from build123d import *

# Parameters (mm, degrees)
BOSS_EXTRUDE2_DEPTH = 6.35
SKETCH2_R           = 3.175
CUT_EXTRUDE1_DEPTH  = 7.35
SKETCH7_R           = 2.286
CUT_EXTRUDE3_DEPTH  = 12.7
SKETCH8_R           = 2.286
CUT_EXTRUDE4_DEPTH  = 7.35
SKETCH9_W           = 129.404437756
SKETCH9_H           = 25.4
CUT_EXTRUDE5_DEPTH  = 7.35
CUT_EXTRUDE6_DEPTH  = 3.175
BOSS_EXTRUDE3_DEPTH = 3.81
CHAMFER1_SIZE       = 2.54


with BuildPart() as part:
    # Sketch1 → Boss-Extrude2 (new body)
    with BuildSketch(Plane(origin=(0, 0, 0), x_dir=(1, 0, 0), z_dir=(0, 1, 0))):
        with BuildLine():
            Line((0, 0), (0, 25.4))
            ThreePointArc((0, 25.4), (3.719743879, 34.380256121), (12.7, 38.1))
            Line((12.7, 38.1), (190.5, 38.1))
            ThreePointArc((190.5, 38.1), (199.480256121, 34.380256121), (203.2, 25.4))
            Line((203.2, 25.4), (203.2, -152.4))
            ThreePointArc((203.2, -152.4), (199.480256121, -161.380256121), (190.5, -165.1))
            Line((190.5, -165.1), (12.7, -165.1))
            ThreePointArc((12.7, -165.1), (3.719743879, -161.380256121), (0, -152.4))
            Line((0, -152.4), (0, -127))
            Line((0, -127), (181.61, -127))
            Line((181.61, -127), (181.61, 0))
            Line((181.61, 0), (0, 0))
        make_face()
    extrude(amount=BOSS_EXTRUDE2_DEPTH)

    # Sketch2 → Cut-Extrude1 (cut, through all)
    with BuildSketch(Plane(origin=(0, 6.35, 0), x_dir=(1, 0, 0), z_dir=(0, 1, 0))):
        with Locations((12.7, 25.4)):
            Circle(SKETCH2_R)
        with Locations((190.5, 25.4)):
            Circle(SKETCH2_R)
        with Locations((190.5, -152.4)):
            Circle(SKETCH2_R)
        with Locations((12.7, -152.4)):
            Circle(SKETCH2_R)
    extrude(amount=-CUT_EXTRUDE1_DEPTH, mode=Mode.SUBTRACT)

    # Sketch7 → Cut-Extrude3 (cut)
    with BuildSketch(Plane(origin=(0, 6.35, 0), x_dir=(1, 0, 0), z_dir=(0, 1, 0))):
        with Locations((192.024, -101.092)):
            Circle(SKETCH7_R)
        with Locations((192.024, -91.186)):
            Circle(SKETCH7_R)
        with Locations((192.024, -35.814)):
            Circle(SKETCH7_R)
        with Locations((192.024, -25.908)):
            Circle(SKETCH7_R)
    extrude(amount=-CUT_EXTRUDE3_DEPTH, mode=Mode.SUBTRACT)

    # Sketch8 → Cut-Extrude4 (cut, through all)
    with BuildSketch(Plane(origin=(0, 0, 0), x_dir=(-1, 0, 0), z_dir=(0, -1, 0))):
        with Locations((-24.197781122, 13.902218878)):
            Circle(SKETCH8_R)
        with Locations((-24.197781122, -140.902218878)):
            Circle(SKETCH8_R)
        with Locations((-179.002218878, -140.902218878)):
            Circle(SKETCH8_R)
        with Locations((-179.002218878, 13.902218878)):
            Circle(SKETCH8_R)
    extrude(amount=-CUT_EXTRUDE4_DEPTH, mode=Mode.SUBTRACT)

    # Sketch9 → Cut-Extrude5 (cut, through all)
    with BuildSketch(Plane(origin=(0, 6.35, 0), x_dir=(1, 0, 0), z_dir=(0, 1, 0))):
        with Locations((101.6, 12.7)):
            Rectangle(SKETCH9_W, SKETCH9_H)
        with Locations((101.6, -139.7)):
            Rectangle(SKETCH9_W, SKETCH9_H)
    extrude(amount=-CUT_EXTRUDE5_DEPTH, mode=Mode.SUBTRACT)

    # Sketch10 → Cut-Extrude6 (cut)
    with BuildSketch(Plane(origin=(0, 6.35, 0), x_dir=(1, 0, 0), z_dir=(0, 1, 0))):
        Polygon((0, 6.35), (30.547781122, 6.35), (30.547781122, 31.75), (172.652218878, 31.75), (172.652218878, 6.35), (181.61, 6.35), (181.61, 0), (166.302218878, 0), (166.302218878, 25.4), (36.897781122, 25.4), (36.897781122, 0), (0, 0), align=None)
        Polygon((0, -127), (0, -133.35), (30.547781122, -133.35), (30.547781122, -158.75), (172.652218878, -158.75), (172.652218878, -133.35), (181.61, -133.35), (181.61, -127), (166.302218878, -127), (166.302218878, -152.4), (36.897781122, -152.4), (36.897781122, -127), align=None)
    extrude(amount=-CUT_EXTRUDE6_DEPTH, mode=Mode.SUBTRACT)

    # Sketch11 → Boss-Extrude3 (add)
    with BuildSketch(Plane.XZ):
        with BuildLine():
            Line((174.07128, -38.1), (187.384850533, -24.786429467))
            ThreePointArc((187.384850533, -24.786429467), (187.552268433, -26.579620112), (188.668154157, -27.993253903))
            Line((188.668154157, -27.993253903), (178.561408061, -38.1))
            Line((178.561408061, -38.1), (174.07128, -38.1))
        make_face()
        with BuildLine():
            Line((203.2, -8.97128), (203.2, -13.461408061))
            Line((203.2, -13.461408061), (193.093253903, -23.568154157))
            ThreePointArc((193.093253903, -23.568154157), (191.679620112, -22.452268433), (189.886429467, -22.284850533))
            Line((189.886429467, -22.284850533), (203.2, -8.97128))
        make_face()
        with BuildLine():
            Line((10.106746097, -23.568154157), (0, -13.461408061))
            Line((0, -13.461408061), (0, -8.97128))
            Line((0, -8.97128), (13.313570533, -22.284850533))
            ThreePointArc((13.313570533, -22.284850533), (11.520379888, -22.452268433), (10.106746097, -23.568154157))
        make_face()
        with BuildLine():
            Line((15.815149467, -24.786429467), (29.12872, -38.1))
            Line((29.12872, -38.1), (24.638591939, -38.1))
            Line((24.638591939, -38.1), (14.531845843, -27.993253903))
            ThreePointArc((14.531845843, -27.993253903), (15.647731567, -26.579620112), (15.815149467, -24.786429467))
        make_face()
        with BuildLine():
            Line((14.531845843, 154.993253903), (24.638591939, 165.1))
            Line((24.638591939, 165.1), (29.12872, 165.1))
            Line((29.12872, 165.1), (15.815149467, 151.786429467))
            ThreePointArc((15.815149467, 151.786429467), (15.647731567, 153.579620112), (14.531845843, 154.993253903))
        make_face()
        with BuildLine():
            Line((13.313570533, 149.284850533), (0, 135.97128))
            Line((0, 135.97128), (0, 140.461408061))
            Line((0, 140.461408061), (10.106746097, 150.568154157))
            ThreePointArc((10.106746097, 150.568154157), (11.520379888, 149.452268433), (13.313570533, 149.284850533))
        make_face()
        with BuildLine():
            Line((193.093253903, 150.568154157), (203.2, 140.461408061))
            Line((203.2, 140.461408061), (203.2, 135.97128))
            Line((203.2, 135.97128), (189.886429467, 149.284850533))
            ThreePointArc((189.886429467, 149.284850533), (191.679620112, 149.452268433), (193.093253903, 150.568154157))
        make_face()
        with BuildLine():
            Line((187.384850533, 151.786429467), (174.07128, 165.1))
            Line((174.07128, 165.1), (178.561408061, 165.1))
            Line((178.561408061, 165.1), (188.668154157, 154.993253903))
            ThreePointArc((188.668154157, 154.993253903), (187.552268433, 153.579620112), (187.384850533, 151.786429467))
        make_face()
    extrude(amount=BOSS_EXTRUDE3_DEPTH)

    # Chamfer1
    chamfer1_edges = [part.edges().sort_by_distance(p)[0] for p in [
        (183.614781109, -3.81, -33.046626952),
        (198.146626952, -3.81, -18.514781109),
        (5.053373048, -3.81, -18.514781109),
        (19.585218891, -3.81, -33.046626952),
        (19.585218891, -3.81, 160.046626952),
        (5.053373048, -3.81, 145.514781109),
        (198.146626952, -3.81, 145.514781109),
        (183.614781109, -3.81, 160.046626952),
    ]]
    chamfer(chamfer1_edges, length=CHAMFER1_SIZE)


solid = part.part
The listing builds one solid part. Answer for the finished solid, in the listing's coordinates (mm). A direction names the side the tool comes from. Coordinates: 2 decimals unless noted, no trailing zeros. Write each loop counter-clockwise with the first axis right and the second up, starting at its lowest first coordinate (ties: lowest second). Pieces come first, ordered by that corner, then holes. Notation, with made-up numbers: (32.5, -30) - (51.5, -30) arc R18 ccw to (51.5, -25) - close; hole circle Ø9 at (34.25, 39.5). An arc over 180 degrees is marked (long way). Put each result on its own line as item: value.
1. Find the intervals of material crossed by line 1 along X through (y, z) = (4.75, -25.4) (3 decimals); line 2 along Z through (x, y) = (92.5, 5); line 3 along Z through (x, y) = (145.5, 1.75), in increasing order. Write a range as from..to.
Answer sheet:
line 1: x = 0..9.525, 15.875..30.548, 172.652..187.325, 193.675..203.2
line 2: z = -38.1..-31.75, 158.75..165.1
line 3: z = -38.1..-25.4, 152.4..165.1
2. The part is cut by section B-B on z = 11. Give the vertices of the cut face in (x, y), plus the area to 3 significant figures.
Answer sheet:
outline: (181.61, 0) - (203.2, 0) - (203.2, 6.35) - (181.61, 6.35) - close
area: 137 mm^2
3. Determine the mould class of faces 1 (the face through (182.15, -2.52, -32.74)), 2 (the face through (198.076, -0.626, 145.586)), 3 (the face through (10, 0, -29)), 4 (the face through (181.61, 3, 64)) for opening direction Z: pulls with the +Z half, pulls with the -Z half, needs draft (parallel to the pull), parting line crosses it, or undercut.
Answer sheet:
face 1: pulls with the -Z half
face 2: pulls with the +Z half
face 3: needs draft
face 4: undercut
4. A tool of negligible diameter and unlimited length cuts with its end or side. For faces 5 (the face through (7, 0, 158)), 6 (the face through (6.56, -1.88, -15.53)), 7 (the face through (183.54, -0.63, 160.12)), from which of +Z, -Z, +X, -X, +Y, -Y can it reach the whole face along a straight path? Write none if from no direction.
Answer sheet:
face 5: +Z, -X, -Y
face 6: -Y
face 7: +Z, +X, -Y
5. The part is cut by section A-A on x = 145.5. Give the vertices of the cut face in (y, z) (3 decimals), plus the area to 3 significant figures.
Answer sheet:
outline: (0, -38.1) - (6.35, -38.1) - (6.35, -31.75) - (3.175, -31.75) - (3.175, -25.4) - (0, -25.4) - close; (0, 152.4) - (3.175, 152.4) - (3.175, 158.75) - (6.35, 158.75) - (6.35, 165.1) - (0, 165.1) - close
area: 121 mm^2
6. Flat-ended cylindrical pins translate along their axes: pin 1 Ø1.5 at (y, z) = (2.5, -10) entering from -X; pin 2 Ø7.5 at (x, z) = (24.2, 140.9) entering from -Y; pin 3 Ø9.5 at (x, z) = (66.5, 143.5) entering from +Y; pin 4 Ø1 at (x, y) = (11, 1) entering from -Z. Find the tip coordinate at first contact, or state that the pin passes through.
Answer sheet:
pin 1: stops at x = 0
pin 2: stops at y = 0
pin 3: passes through
pin 4: stops at z = -38.04
